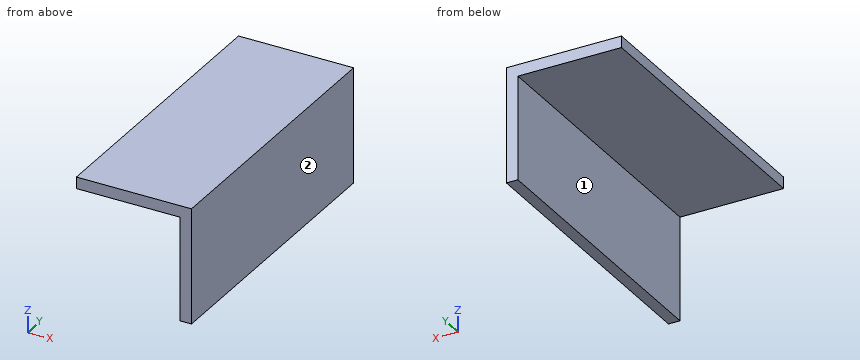
Autodesk Inventor part; units mm, degrees
ref_plane "YZ Plane" through (0, 0, 0) normal (1, 0, 0) x (0, 1, 0)
ref_plane "XZ Plane" through (0, 0, 0) normal (0, 1, 0) x (-1, 0, 0)
ref_plane "XY Plane" through (0, 0, 0) normal (0, 0, 1) x (1, 0, 0)
sketch "Sketch1" plane through (0, 0, 0) normal (0, 1, 0) x (-1, 0, 0)
  line L0 (0, 0) -> (5.08, 0)
  line L1 (5.08, 0) -> (5.08, 50.8)
  line L2 (5.08, 50.8) -> (0, 50.8)
  line L3 (0, 50.8) -> (0, 0)
  line L4 (5.08, 50.8) -> (50.8, 50.8)
  line L5 (50.8, 50.8) -> (50.8, 45.72)
  line L6 (50.8, 45.72) -> (5.08, 45.72)
  line L7 (5.08, 45.72) -> (5.08, 50.8)
  point P0 (5.08, 45.72)
  dimension "d5" = 50.8
  dimension "d6" = 5.08
  dimension "d7" = 5.08
  dimension "d8" = 50.8
extrude "Extrusion1" add sketch "Sketch1" along normal blind 127
properties part number "Flower Box Stack Half"
Part model, mm, in its own coordinate system. Face numbers are marked on the shaded views. A direction names the side the tool comes from. Coordinates: 2 decimals unless noted, no trailing zeros. Order: outer loops, then holes, each group sorted by start corner. A loop starts at its lowest first (then second) coordinate and runs counter-clockwise, first axis right, second up. Notation, with made-up numbers: (72, 64) -> (79, 64) arc R29 ccw to (79, 103) -> close; hole circle Ø3 at (11.25, 50). An arc over 180 degrees is marked (long way). Put each result on its own line as item: value. Start each with the question number.
(1) Band-saw the part on C-C (x = -41.5). Give the cut face in (y, z).
(2) Probe line 1 along X through (y, z) = (113, 24); line 2 along Z through (x, y) = (-19, 87). List the from-to ranges inside material, lowest first. Write a range as [from, to].
(3) Pin check, flat tips, straight feed: pin 1 Ø2 at (y, z) = (68.5, 21.5) entering from -X; pin 2 Ø3 at (x, y) = (-43, 59.5) entering from -Z. Stop position of each tip, or through.
(4) Which spindle directions (+Z, -Z, +X, -X, +Y, -Y) get a long thin tool onto all of the face, cutting with end or side? Do the marked faces 1 and 2. Say none if no direction does.
(5) Band-saw the part on B-B (z = 10.5). Give the cut face in (x, y).
(6) Band-saw the part on A-A (y = 103). Give the cut face in (x, z), then the cut area to 3 significant figures.
Determined:
1. outline: (0, 45.72) -> (127, 45.72) -> (127, 50.8) -> (0, 50.8) -> close
2. line 1: x = [-5.08, 0]
2. line 2: z = [45.72, 50.8]
3. pin 1: stops at x = -5.08
3. pin 2: stops at z = 45.72
4. face 1: -Z, -X, +Y, -Y
4. face 2: +Z, -Z, +X, +Y, -Y
5. outline: (-5.08, 0) -> (0, 0) -> (0, 127) -> (-5.08, 127) -> close
6. outline: (-50.8, 45.72) -> (-5.08, 45.72) -> (-5.08, 0) -> (0, 0) -> (0, 50.8) -> (-50.8, 50.8) -> close
6. area: 490 mm²
